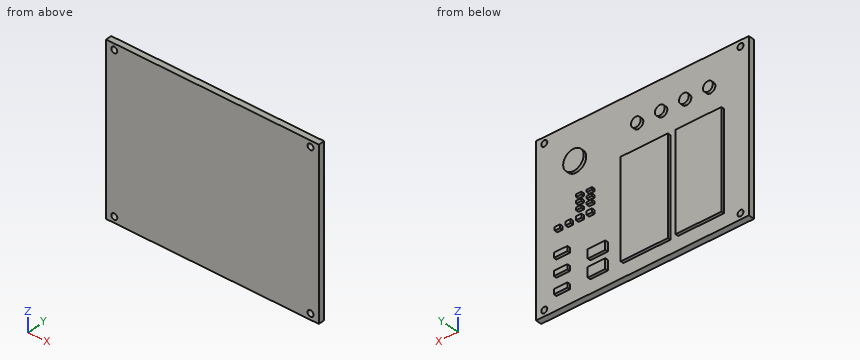
from build123d import *

# Parameters (mm, degrees)
SKETCH1_W               = 90
SKETCH1_H               = 70
BOSS_EXTRUDE1_DEPTH     = 2.54
SKETCH2_R               = 2.074775273
SKETCH2_R_2             = 4.325167344
SKETCH2_W               = 2.219761911
SKETCH2_H               = 1.524543627
SKETCH2_W_2             = 19.349952437
SKETCH2_H_2             = 40.787411984
SKETCH2_W_3             = 19.977857201
SKETCH2_W_4             = 7.399206371
SKETCH2_H_3             = 4.17028531
SKETCH2_H_4             = 3.699603186
SKETCH2_W_5             = 5.771380969
SKETCH2_H_5             = 2.032
SKETCH2_H_6             = 1.035888892
SKETCH2_W_6             = 2.219761912
SKETCH2_H_7             = 1.578831572
SKETCH2_H_8             = 1.553833338
SKETCH2_H_9             = 1.493763587
BOSS_EXTRUDE2_DEPTH     = 1.27
SKETCH3_R               = 1.27
CUT_EXTRUDE1_DEPTH      = 2.54
MIRROR2_COPY_1_SKETCH_R = 1.27
MIRROR2_COPY_1_DEPTH    = 2.54


with BuildPart() as part:
    # Sketch1 → Boss-Extrude1 (new body)
    with BuildSketch(Plane(origin=(0, 0, 0), x_dir=(1, 0, 0), z_dir=(0, 1, 0))):
        Rectangle(SKETCH1_W, SKETCH1_H)
    extrude(amount=BOSS_EXTRUDE1_DEPTH)

    # Sketch2 → Boss-Extrude2 (add)
    with BuildSketch(Plane(origin=(0, 2.54, 0), x_dir=(1, 0, 0), z_dir=(0, 1, 0))):
        with Locations(Location((-28.787636227, -22.056380876, 0), (0, 0, 270))):
            Circle(SKETCH2_R)
        with Locations(Location((-18.627636227, -22.056380876, 0), (0, 0, 270))):
            Circle(SKETCH2_R)
        with Locations(Location((-8.467636227, -22.056380876, 0), (0, 0, 270))):
            Circle(SKETCH2_R)
        with Locations(Location((1.692363773, -22.056380876, 0), (0, 0, 270))):
            Circle(SKETCH2_R)
        with Locations(Location((28.076508074, -19.269666276, 0), (0, 0, 270))):
            Circle(SKETCH2_R_2)
        with Locations((30.364354819, 3.966137277)):
            Rectangle(SKETCH2_W, SKETCH2_H)
        with Locations((-24.784583824, 8.975791822)):
            Rectangle(SKETCH2_W_2, SKETCH2_H_2)
        with Locations((-1.882735108, 8.975791822)):
            Rectangle(SKETCH2_W_3, SKETCH2_H_2)
        with Locations((18.317098286, 27.284355159)):
            Rectangle(SKETCH2_W_4, SKETCH2_H_3)
        with Locations((18.317098286, 20.093760108)):
            Rectangle(SKETCH2_W_4, SKETCH2_H_4)
        with Locations((33.485471346, 28.353497814)):
            Rectangle(SKETCH2_W_5, SKETCH2_H_5)
        with Locations((33.485471346, 21.241497814)):
            Rectangle(SKETCH2_W_5, SKETCH2_H_5)
        with Locations((33.485471346, 14.129497814)):
            Rectangle(SKETCH2_W_5, SKETCH2_H_5)
        with Locations((21.352830995, 0.193252065)):
            Rectangle(SKETCH2_W, SKETCH2_H_6)
        with Locations((25.858592907, 3.938993304)):
            Rectangle(SKETCH2_W_6, SKETCH2_H_7)
        with Locations((21.352830995, 3.951492421)):
            Rectangle(SKETCH2_W, SKETCH2_H_8)
        with Locations((34.870116729, 3.981527297)):
            Rectangle(SKETCH2_W, SKETCH2_H_9)
        with Locations((21.352830995, -2.195488046)):
            Rectangle(SKETCH2_W, SKETCH2_H_6)
        with Locations((21.352830995, -4.651515111)):
            Rectangle(SKETCH2_W, SKETCH2_H_6)
        with Locations((25.858592907, 0.289779343)):
            Rectangle(SKETCH2_W_6, SKETCH2_H_6)
        with Locations((25.858592907, -2.300212834)):
            Rectangle(SKETCH2_W_6, SKETCH2_H_6)
        with Locations((25.858592907, -4.890205011)):
            Rectangle(SKETCH2_W_6, SKETCH2_H_6)
    extrude(amount=BOSS_EXTRUDE2_DEPTH)

    # Sketch3 → Cut-Extrude1 (cut)
    with BuildSketch(Plane(origin=(0, 2.54, 0), x_dir=(1, 0, 0), z_dir=(0, 1, 0))):
        with Locations(Location((-41.49861, 32.4854, 0), (0, 0, 270))):
            Circle(SKETCH3_R)
    cut_extrude1 = extrude(amount=-CUT_EXTRUDE1_DEPTH, mode=Mode.SUBTRACT)

    # Mirror1: Cut-Extrude1 across plane
    add(cut_extrude1.mirror(Plane(origin=(0, 0, 0), x_dir=(1, 0, 0), z_dir=(0, 0, -1))), mode=Mode.SUBTRACT)

    # Mirror2: Cut-Extrude1 across plane
    add(cut_extrude1.mirror(Plane.ZY), mode=Mode.SUBTRACT)

    # Mirror2 copy 1 sketch → Mirror2 copy 1 (cut)
    with BuildSketch(Plane(origin=(0, 2.54, 0), x_dir=(-1, 0, 0), z_dir=(0, 1, 0))):
        with Locations(Location((-41.49861, 32.4854, 0), (0, 0, 270))):
            Circle(MIRROR2_COPY_1_SKETCH_R)
    extrude(amount=-MIRROR2_COPY_1_DEPTH, mode=Mode.SUBTRACT)


solid = part.part
Could you check a few things on this model? Use its own coordinates, in mm. Coordinates: 2 decimals unless noted, no trailing zeros. Write each loop counter-clockwise with the first axis right and the second up, starting at its lowest first coordinate (ties: lowest second). Pieces come first, ordered by that corner, then holes. Notation, with made-up numbers: (10, 78) - (37, 78) arc R15 ccw to (37, 89) - close; hole circle Ø4 at (88.5, 55.25). An arc over 180 degrees is marked (long way). Write item = value, one per line.
1) Suppose I cut it at A-A on x = -23. Please give me the cut outline in (y, z), plus the area to 3 significant figures.
Result set:
outline = (0, -35) - (2.54, -35) - (2.54, -29.37) - (3.81, -29.37) - (3.81, 11.42) - (2.54, 11.42) - (2.54, 35) - (0, 35) - close
area = 230 mm2
2) Please list where these lines run through material, in increasing order: line 1 (X direction, y = 3.55, z = -7.5); line 2 (X direction, y = 2.2, z = -32); line 3 (Y direction, x = -17, z = 31). Write a range as [from, to].
Result set:
line_1 = [-34.46, -15.11], [-11.87, 8.11]
line_2 = [-45, -42.67], [-40.33, 40.33], [42.67, 45]
line_3 = [0, 2.54]
3) Suppose I cut it at B-B on z = 28.5. Please give me the cut outline in (x, y).
Result set:
outline = (-45, 0) - (45, 0) - (45, 2.54) - (-45, 2.54) - close
4) Suppose I cut it at C-C on x = 11. Please give me the cut outline in (y, z), plus the area to 3 significant figures.
Result set:
outline = (0, -35) - (2.54, -35) - (2.54, 35) - (0, 35) - close
area = 178 mm2
5) Will these pins go through, and if not, where does the flat tip stop? pin 1 Ø0.6 at (x, y) = (26, 3) entering from -Z; pin 2 Ø1 at (y, z) = (3.5, -4) entering from +X; pin 3 Ø0.6 at (x, y) = (21.5, 3.5) entering from +Z.
Result set:
pin_1 = -4.73
pin_2 = 35.98
pin_3 = 5.17
